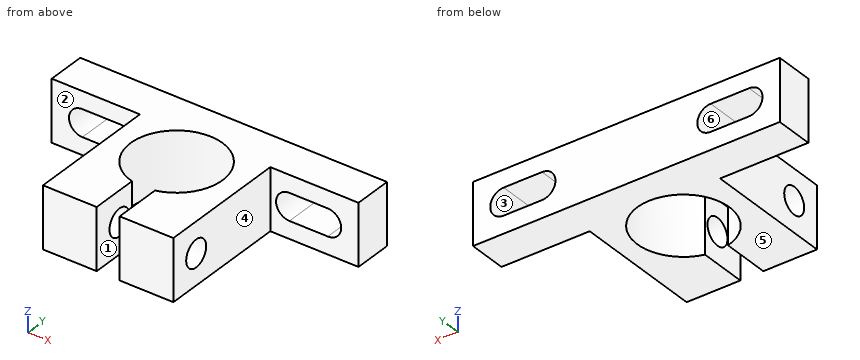
```python
from build123d import *

# Parameters (mm, degrees)
EXTRUDE_1_DEPTH     = 8
CUT_EXTRUDE_1_DEPTH = 8
SKETCH_3_R          = 1.75
CUT_EXTRUDE_2_DEPTH = 26


with BuildPart() as part:
    # 草图1 → 凸台-拉伸1 (new body)
    with BuildSketch(Plane.XY):
        with BuildLine():
            Line((20, 10), (-20, 10))
            Line((-20, 10), (-20, 5))
            Line((-20, 5), (-8.5, 5))
            Line((-8.5, 5), (-8.5, -12))
            Line((-8.5, -12), (-1.5, -12))
            Line((-1.5, -12), (-1.5, -5.809475019))
            ThreePointArc((-1.5, -5.809475019), (0, 6), (1.5, -5.809475019))
            Line((1.5, -5.809475019), (1.5, -12))
            Line((1.5, -12), (8.5, -12))
            Line((8.5, -12), (8.5, 5))
            Line((8.5, 5), (20, 5))
            Line((20, 5), (20, 10))
        make_face()
    extrude(amount=EXTRUDE_1_DEPTH)

    # 草图2 → 切除-拉伸1 (cut)
    with BuildSketch(Plane(origin=(0, 10, 0), x_dir=(1, 0, 0), z_dir=(0, 1, 0))):
        with BuildLine():
            Line((-16, -2.25), (-11, -2.25))
            ThreePointArc((-11, -2.25), (-9.25, -4), (-11, -5.75))
            Line((-11, -5.75), (-16, -5.75))
            ThreePointArc((-16, -5.75), (-17.75, -4), (-16, -2.25))
        make_face()
        with BuildLine():
            Line((16, -5.75), (11, -5.75))
            ThreePointArc((11, -5.75), (9.25, -4), (11, -2.25))
            Line((11, -2.25), (16, -2.25))
            ThreePointArc((16, -2.25), (17.75, -4), (16, -5.75))
        make_face()
    extrude(amount=-CUT_EXTRUDE_1_DEPTH, mode=Mode.SUBTRACT)

    # 草图3 → 切除-拉伸2 (cut)
    with BuildSketch(Plane.ZY.offset(8.5)):
        with Locations((4, -8)):
            Circle(SKETCH_3_R)
    extrude(amount=-CUT_EXTRUDE_2_DEPTH, mode=Mode.SUBTRACT)


solid = part.part
```
Design review of the part built by this model. Coordinates are the model's own, in mm. Face numbers are marked on the shaded views. A direction names the side the tool comes from. Coordinates: 2 decimals unless noted, no trailing zeros. Order: outer loops, then holes, each group sorted by start corner. A loop starts at its lowest first (then second) coordinate and runs counter-clockwise, first axis right, second up. Notation, with made-up numbers: M 42.25,58.25 L 75.25,58.25 A7 ccw 75.25,68.25 Z; hole C 80.5,50 d11. An arc over 180 degrees is marked long. Answer as a JSON object with one key per item and string values. Group by question number.
1) For pin 1 (2.5 mm diameter, centred on x = 14, z = 3, fed in from -Y); pin 2 (3 mm diameter, centred on y = -9, z = 5, fed in from +X); pin 3 (2 mm diameter, centred on y = -8, z = 4, fed in from -X); pin 4 (3 mm diameter, centred on y = -8, z = 3.5, fed in from -X), all flat-tipped, find the tip position at first contact; note any pin that passes through.
2) Mouldability with a two-part tool opening along Z and no side actions: class the marked faces 4, 5 and 6 as pulls with the +Z half, pulls with the -Z half, needs draft (parallel to the pull), parting line crosses it, or undercut.
3) Add section D-D, the plane x = -3.5. Write out the cut boundary in (y, z).
4) Add section A-A, the plane y = 0. Write out the cut boundary in (x, z).
5) Add section B-B, the plane y = -8. Write out the cut boundary in (x, z), then the cut area to 3 significant figures.
6) Tool access review of the marked faces 1, 2 and 3: name each direction out of +Z, -Z, +X, -X, +Y, -Y from which nothing blocks a thin tool from reaching the whole face with its end or side.
7) Add section C-C, the plane z = 4. Write out the cut boundary in (x, y), then the cut area to 3 significant figures.
8) Wall thickness on L1, parallel to X at y = -6.5, z = 3; L2, parallel to Y at x = 2.5, z = 4.25; L3, parallel to Y at x = -3.75, z = 4: over which ranges is each line inside the solid? List them lowest first.
Computed values:
{
 "1": {"pin 1": "stops at y = 5", "pin 2": "stops at x = 8.5", "pin 3": "passes through", "pin 4": "stops at x = -8.5"},
 "2": {"face 4": "needs draft", "face 5": "pulls with the -Z half", "face 6": "undercut"},
 "3": {"outline": "M -12,0 L -4.87,0 L -4.87,8 L -12,8 Z; M 4.87,0 L 10,0 L 10,8 L 4.87,8 Z; hole C -8,4 d3.5"},
 "4": {"outline": "M -8.5,0 L -6,0 L -6,8 L -8.5,8 Z; M 6,0 L 8.5,0 L 8.5,8 L 6,8 Z"},
 "5": {"outline": "M -8.5,0 L -1.5,0 L -1.5,2.25 L -8.5,2.25 Z; M -8.5,5.75 L -1.5,5.75 L -1.5,8 L -8.5,8 Z; M 1.5,0 L 8.5,0 L 8.5,2.25 L 1.5,2.25 Z; M 1.5,5.75 L 8.5,5.75 L 8.5,8 L 1.5,8 Z", "area": "63.0 mm^2"},
 "6": {"face 1": "+Z, -Z, -Y", "face 2": "+Z, -Z, -X, -Y", "face 3": "+Y, -Y"},
 "7": {"outline": "M -20,5 L -17.75,5 L -17.75,10 L -20,10 Z; M -9.25,5 L -8.5,5 L -8.5,-6.25 L -1.5,-6.25 L -1.5,-5.81 A6 cw long 1.5,-5.81 L 1.5,-6.25 L 8.5,-6.25 L 8.5,5 L 9.25,5 L 9.25,10 L -9.25,10 Z; M -8.5,-12 L -1.5,-12 L -1.5,-9.75 L -8.5,-9.75 Z; M 1.5,-12 L 8.5,-12 L 8.5,-9.75 L 1.5,-9.75 Z; M 17.75,5 L 20,5 L 20,10 L 17.75,10 Z", "area": "224 mm^2"},
 "8": {"L1": "x = -8.5 to -1.5, 1.5 to 8.5", "L2": "y = -12 to -9.73, -6.27 to -5.45, 5.45 to 10", "L3": "y = -12 to -9.75, -6.25 to -4.68, 4.68 to 10"}
}
